from build123d import *

# Parameters (mm, degrees)
SKETCH1_R           = 2.38125
BOSS_EXTRUDE1_DEPTH = 3.175


with BuildPart() as part:
    # Sketch1 → Boss-Extrude1 (new body)
    with BuildSketch(Plane(origin=(0, 0, 0), x_dir=(1, 0, 0), z_dir=(0, 1, 0))):
        with BuildLine():
            ThreePointArc((0, 2.54), (0.743948776, 0.743948776), (2.54, 0))
            Line((2.54, 0), (25.4, 0))
            Line((25.4, 0), (73.66, 0))
            ThreePointArc((73.66, 0), (75.456051224, 0.743948776), (76.2, 2.54))
            Line((76.2, 2.54), (76.2, 22.86))
            ThreePointArc((76.2, 22.86), (75.456051224, 24.656051224), (73.66, 25.4))
            Line((73.66, 25.4), (27.94, 25.4))
            ThreePointArc((27.94, 25.4), (26.143948776, 26.143948776), (25.4, 27.94))
            Line((25.4, 27.94), (25.4, 73.66))
            ThreePointArc((25.4, 73.66), (24.656051224, 75.456051224), (22.86, 76.2))
            Line((22.86, 76.2), (2.54, 76.2))
            ThreePointArc((2.54, 76.2), (0.743948776, 75.456051224), (0, 73.66))
            Line((0, 73.66), (0, 25.4))
            Line((0, 25.4), (0, 2.54))
        make_face()
        with Locations((12.7, 12.7)):
            Circle(SKETCH1_R, mode=Mode.SUBTRACT)
        with Locations((25.4, 12.7)):
            Circle(SKETCH1_R, mode=Mode.SUBTRACT)
        with Locations((38.1, 12.7)):
            Circle(SKETCH1_R, mode=Mode.SUBTRACT)
        with Locations((12.7, 25.4)):
            Circle(SKETCH1_R, mode=Mode.SUBTRACT)
        with Locations((12.7, 38.1)):
            Circle(SKETCH1_R, mode=Mode.SUBTRACT)
        with Locations((50.8, 12.7)):
            Circle(SKETCH1_R, mode=Mode.SUBTRACT)
        with Locations((63.5, 12.7)):
            Circle(SKETCH1_R, mode=Mode.SUBTRACT)
        with Locations((12.7, 50.8)):
            Circle(SKETCH1_R, mode=Mode.SUBTRACT)
        with Locations((12.7, 63.5)):
            Circle(SKETCH1_R, mode=Mode.SUBTRACT)
    extrude(amount=BOSS_EXTRUDE1_DEPTH)


solid = part.part
Read the model definition and answer for the solid it produces. Units are mm, in the model's axes. A direction names the side the tool comes from. Give positions to 0.01 mm unless a question says otherwise; leave off trailing zeros. Write each loop counter-clockwise with the first axis right and the second up, starting at its lowest first coordinate (ties: lowest second). Pieces come first, ordered by that corner, then holes. Notation, with made-up numbers: (30.5, 21.5) -> (78.5, 21.5) arc R18 ccw to (78.5, 49.5) -> close; hole circle Ø3 at (69, 62.5). An arc over 180 degrees is marked (long way). Answer as a JSON object with one key per item and string values. Group by question number.
1) Find section C-C (y = 0.9). Count the separate pieces of the cut face and the enclosed holes in it, and give its area (3 significant figures).
2) Each of these flat-tipped pins is pushed along its axis until it touches: P1, Ø1, axis at y = 1.5, z = -44, coming from the +X side; P2, Ø3, axis at x = 50.8, z = -12.7, coming from the -Y side. Where does it stop, or does it pass through?
3) Find section B-B (z = -38.1). Write down the section's boundary in (x, y) (3 decimals), and give its area (3 significant figures).
4) The mould has two halves that part along Z. Classify faces 3 (the cylindrical face through (13.98, 1.57, -14.71)), 4 (the cylindrical face through (24.676, 1.565, -75.436)), 5 (the flat face through (0, 2, -39)): +Z half, -Z half, draft (parallel to the pull), parting line (faces both ways), or undercut.
5) Consider L1, parallel to X at y = 0.85, z = -12.7; L2, parallel to Z at x = 12.7, y = 1.7; L3, parallel to Z at x = 50.8, y = 2.1. Determine where each line is inside the solid, lowest interval first. Write a range as from..to.
6) A tool of negligible diameter and unlimited length cuts with its end or side. For faces 1 (the flat face through (51, 2, -25.4)), 2 (the cylindrical face through (40.37, 1.57, -13.42)), from which of +Z, -Z, +X, -X, +Y, -Y can it reach the whole face along a straight path? Write none if from no direction.
7) Find section A-A (x = 50.8). Write down the section's boundary in (y, z) (3 decimals), and give its area (3 significant figures).
8) Find section D-D (x = 12.7). Write down the section's boundary in (y, z) (3 decimals), and give its area (3 significant figures).
Values follow:
{
 "1": {"separate pieces": "1", "enclosed holes": "9", "area": "3,060 mm2"},
 "2": {"P1": "stops at x = 25.4", "P2": "passes through"},
 "3": {"outline": "(0, 0) -> (10.319, 0) -> (10.319, 3.175) -> (0, 3.175) -> close; (15.081, 0) -> (25.4, 0) -> (25.4, 3.175) -> (15.081, 3.175) -> close", "area": "65.5 mm2"},
 "4": {"face 3": "undercut", "face 4": "-Z half", "face 5": "draft"},
 "5": {"L1": "x = 0..10.32, 15.08..23.02, 27.78..35.72, 40.48..48.42, 53.18..61.12, 65.88..76.2", "L2": "z = -76.2..-65.88, -61.12..-53.18, -48.42..-40.48, -35.72..-27.78, -23.02..-15.08, -10.32..0", "L3": "z = -25.4..-15.08, -10.32..0"},
 "6": {"face 1": "-Z, +X, +Y, -Y", "face 2": "+Y, -Y"},
 "7": {"outline": "(0, -25.4) -> (3.175, -25.4) -> (3.175, -15.081) -> (0, -15.081) -> close; (0, -10.319) -> (3.175, -10.319) -> (3.175, 0) -> (0, 0) -> close", "area": "65.5 mm2"},
 "8": {"outline": "(0, -76.2) -> (3.175, -76.2) -> (3.175, -65.881) -> (0, -65.881) -> close; (0, -61.119) -> (3.175, -61.119) -> (3.175, -53.181) -> (0, -53.181) -> close; (0, -48.419) -> (3.175, -48.419) -> (3.175, -40.481) -> (0, -40.481) -> close; (0, -35.719) -> (3.175, -35.719) -> (3.175, -27.781) -> (0, -27.781) -> close; (0, -23.019) -> (3.175, -23.019) -> (3.175, -15.081) -> (0, -15.081) -> close; (0, -10.319) -> (3.175, -10.319) -> (3.175, 0) -> (0, 0) -> close", "area": "166 mm2"}
}
